Input: part model. Units: mm. Frame: model coordinates. Face numbers are marked on the shaded views. A direction names the side the tool comes from. Round coordinates to 2 decimals unless told otherwise and drop trailing zeros. One line per item, written item: value. Start each with the question number.
from build123d import *

# Parameters (mm, degrees)
BOSS_EXTRUDE1_DEPTH = 5
BOSS_EXTRUDE2_DEPTH = 30
BOSS_EXTRUDE2_TAPER = 10


with BuildPart() as part:
    # Sketch1 → Boss-Extrude1 (new body)
    with BuildSketch(Plane(origin=(0, 0, 0), x_dir=(1, 0, 0), z_dir=(0, 1, 0))):
        with BuildLine():
            Line((-55, 70), (55, 70))
            ThreePointArc((55, 70), (83.284271247, 58.284271247), (95, 30))
            Line((95, 30), (95, -30))
            ThreePointArc((95, -30), (83.284271247, -58.284271247), (55, -70))
            Line((55, -70), (-55, -70))
            ThreePointArc((-55, -70), (-83.284271247, -58.284271247), (-95, -30))
            Line((-95, -30), (-95, 30))
            ThreePointArc((-95, 30), (-83.284271247, 58.284271247), (-55, 70))
        make_face()
    extrude(amount=BOSS_EXTRUDE1_DEPTH)

    # Sketch1_4 → Boss-Extrude2 (add)
    with BuildSketch(Plane(origin=(0, 0, 0), x_dir=(1, 0, 0), z_dir=(0, 1, 0))):
        with BuildLine():
            Line((-55, -60), (55, -60))
            ThreePointArc((55, -60), (76.213203436, -51.213203436), (85, -30))
            Line((85, -30), (85, 30))
            ThreePointArc((85, 30), (76.213203436, 51.213203436), (55, 60))
            Line((55, 60), (-55, 60))
            ThreePointArc((-55, 60), (-76.213203436, 51.213203436), (-85, 30))
            Line((-85, 30), (-85, -30))
            ThreePointArc((-85, -30), (-76.213203436, -51.213203436), (-55, -60))
        make_face()
    extrude(amount=-BOSS_EXTRUDE2_DEPTH, taper=BOSS_EXTRUDE2_TAPER)


solid = part.part
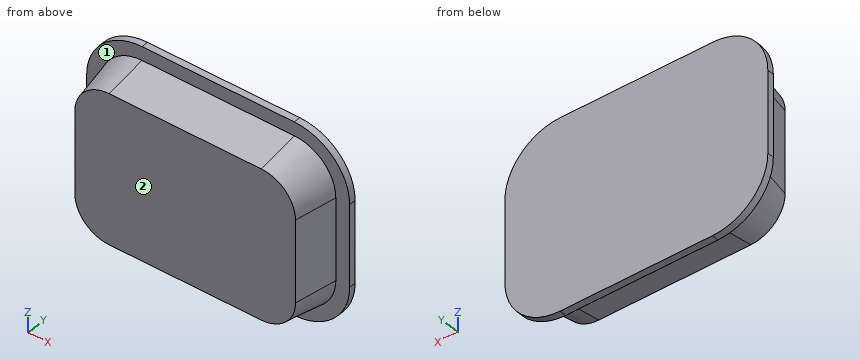
Item 1: Line query: L1, parallel to Y at x = -26, z = -62; L2, parallel to Z at x = -60, y = -25.5; L3, parallel to X at y = 1, z = -56.5. Output: solid intervals per line, ascending.
Item 2: First-contact query: pin 1 Ø8 at (x, y) = (71.5, -2) entering from +Z; pin 2 Ø12 at (x, y) = (67, -0.5) entering from +Z; pin 3 Ø3 at (y, z) = (-18, 36) entering from +X. Flat tips, straight axial feed; report the tip coordinate or a pass-through.
Item 3: Reachability of the marked faces 1 and 2 from +Z, -Z, +X, -X, +Y, -Y: full face, straight path, thin tool, end or side. Return the list, or none.
Geometry results:
1. L1: y = 0 to 5
1. L2: z = -55.01 to 55.01
1. L3: x = -84.96 to 84.96
2. pin 1: stops at z = 67.82
2. pin 2: stops at z = 69.54
2. pin 3: stops at x = 81.56
3. face 1: -Y
3. face 2: +Z, -Z, +X, -X, -Y
